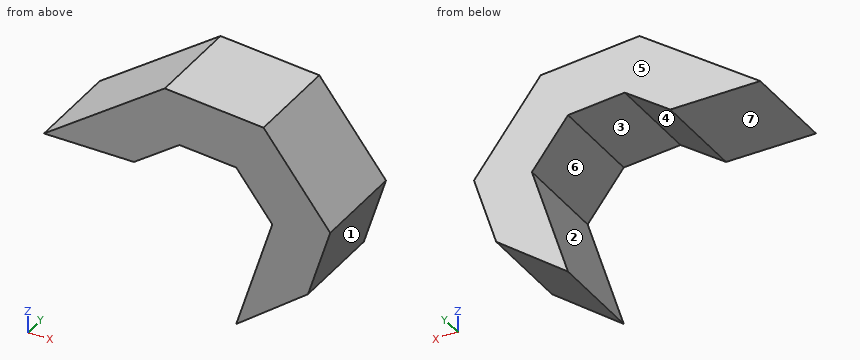
```python
from build123d import *

# Parameters (mm, degrees)
F0_W = 55.5998794734
F0_H = 59.3593008816


with BuildPart() as f2:
    # F2: sweep along a path in F1
    with BuildLine(Plane.XZ) as f2_path:
        Line((0, 0), (51.3951145113, 36.5762151778))
        Line((51.3951145113, 36.5762151778), (99.4288995862, 32.5775817037))
        Line((99.4288995862, 32.5775817037), (131.1959028244, -8.7538054213))
        Line((131.1959028244, -8.7538054213), (113.1796464324, -65.9180954099))
    # F0 (on Top) → F2 (sweep)
    with BuildSketch(Plane.XY):
        Rectangle(F0_W, F0_H)
    sweep(path=f2_path.line, transition=Transition.RIGHT)


solid = f2.part
```
The listing builds one solid part. Answer for the finished solid, in the listing's coordinates (mm). Face numbers are marked on the shaded views. A direction names the side the tool comes from. Coordinates: 2 decimals unless noted, no trailing zeros. Loops run counter-clockwise (first coordinate to the right, second up) from the corner with the lowest first, then second, coordinate; pieces in that order, holes last. Notation, with made-up numbers: M 37,76 L 53,76 A15 cw 53,102 Z; hole C 15.25,89.5 d7. An arc over 180 degrees is marked long. Answer as CSV lines item,"result". Start each with the question number.
(1) Given pin 1 (8 mm diameter, centred on y = -21.5, z = -23, fed in from -X); pin 2 (2 mm diameter, centred on x = 116, y = -3.5, fed in from -Z); pin 3 (5 mm diameter, centred on x = 23.5, y = -22, fed in from -Z), each flat-ended and moving along its own axis, determine where each tip first touches the part or whether it passes through.
(2) The part is cut by section C-C (z = 23). Give the vertices of the cut face in (x, y).
(3) The part is cut by section A-A (y = 10.5). Give the vertices of the cut face in (x, z).
(4) For the marked faces 5, 6 and 7, determine the directions among +Z, -Z, +X, -X, +Y, -Y from which every point of the face is accessible in a straight line to the end or side of a thin tool.
(5) The part is cut by section B-B (x = 38.5). Give the vertices of the cut face in (y, z).
(6) The mould has two halves that part along X. Classify the marked faces 1, 2, 3 and 4: pulls with the +X half, pulls with the -X half, needs draft (parallel to the pull), parting line crosses it, or undercut.
(7) Find the intervals of material crossed by L1, parallel to X at y = 2.5, z = 16; L2, parallel to X at y = -2.5, z = -42.5; L3, parallel to X at y = 2, z = 24, in increasing order. Write a range as [from, to].
Determined:
1,pin 1,"x = 108.54"
1,pin 2,"z = -64.54"
1,pin 3,"z = 0"
2,outline,"M 4.52,-29.68 L 127.12,-29.68 L 127.12,29.68 L 4.52,29.68 Z"
3,outline,"M -27.8,0 L 27.8,0 L 55.94,20.02 L 90.99,17.11 L 113.3,-11.92 L 91,-82.68 L 135.36,-49.16 L 149.09,-5.59 L 107.87,48.05 L 46.85,53.13 Z"
4,face 5,"+Z, -Z, +X, -X, +Y"
4,face 6,"+Y, -Y"
4,face 7,"-Z, -X, +Y, -Y"
5,outline,"M -29.68,7.61 L 29.68,7.61 L 29.68,47.18 L -29.68,47.18 Z"
6,face 1,"pulls with the +X half"
6,face 2,"pulls with the -X half"
6,face 3,"undercut"
6,face 4,"undercut"
7,L1,"[-5.32, 50.28], [91.84, 132.5]"
7,L2,"[103.66, 137.46]"
7,L3,"[5.92, 126.35]"
